from build123d import *

# Parameters (mm, degrees)
F0_R     = 11
F0_R_2   = 9.25
F1_DEPTH = 10
F3_DEPTH = 6
F4_SIZE  = 0.99999


# Not quite as in the source:
# - a fillet or chamfer is up to 0.001 mm smaller than in the source, because OpenCascade refuses the exact size


with BuildPart() as f1:
    # F0 (on Top) → F1 (new body)
    with BuildSketch(Plane.XY):
        Circle(F0_R)
        Circle(F0_R_2, mode=Mode.SUBTRACT)
    extrude(amount=F1_DEPTH)

    # F2 (on face) → F3 (cut)
    with BuildSketch(Plane.XY.offset(10)):
        with BuildLine():
            Line((-10, -4.582575695), (-10, 4.582575695))
            ThreePointArc((-10, 4.582575695), (-11, 0), (-10, -4.582575695))
        make_face()
        with BuildLine():
            ThreePointArc((11, 0), (10.7470926301, 2.3452078799), (10, 4.582575695))
            Line((10, 4.582575695), (10, -4.582575695))
            ThreePointArc((10, -4.582575695), (10.7470926301, -2.3452078799), (11, 0))
        make_face()
    extrude(amount=-F3_DEPTH, mode=Mode.SUBTRACT)

    # F4 (size 1 in the source; OpenCascade refuses exactly that, so slightly less here)
    f4_edges = [f1.edges().sort_by_distance(p)[0] for p in [
        (-11, 0, 0),
        (0, -11, 10),
        (0, 11, 10),
    ]]
    chamfer(f4_edges, length=F4_SIZE)


solid = f1.part
Build history of the part. All positions in model axes, mm. A direction names the side the tool comes from. Round coordinates to 2 decimals unless told otherwise and drop trailing zeros. Write each loop counter-clockwise with the first axis right and the second up, starting at its lowest first coordinate (ties: lowest second). Pieces come first, ordered by that corner, then holes. Notation, with made-up numbers: M 2,69 L 32,69 A23 cw 32,106 Z; hole C 25,74.5 d10. An arc over 180 degrees is marked long. Answer in a Markdown table with one row per item.
1. Saw through at A-A (z = 6.25). List the corners of the cut face in (x, y).
Geometry check:
| item | result |
|---|---|
| outline | M -10,-4.58 A11 ccw 10,-4.58 L 10,4.58 A11 ccw -10,4.58 Z; hole C 0,0 d18.5 |
2. Which spindle directions (+Z, -Z, +X, -X, +Y, -Y) get a long thin tool onto all of the face, cutting with end or side? Do faces 5 (the face through (-11, 0, 3)), 6 (the face through (10, 0, 7)), 7 (the face through (-10.4, 0.1, 4)). Say none if no direction does.
Geometry check:
| item | result |
|---|---|
| face 5 | +Z, -Z |
| face 6 | +Z, +X, +Y, -Y |
| face 7 | +Z, -X, +Y, -Y |
3. Probe L1, parallel to Y at x = 0, z = 6; L2, parallel to Y at x = 2.5, z = 8.5; L3, parallel to X at y = 1.75, z = 0.5. List the from-to ranges inside material, lowest first. Write a range as [from, to].
Geometry check:
| item | result |
|---|---|
| L1 | [-11, -9.25], [9.25, 11] |
| L2 | [-10.71, -8.91], [8.91, 10.71] |
| L3 | [-10.35, -9.08], [9.08, 10.35] |
4. Mould opens along X. For faces 1 (the face through (-0.2, -10.2, 9.8)), 2 (the face through (-10, 0, 7)), 3 (the face through (9, -3, 10)), 4 (the face through (-2.01, -9.03, 4.93)) say: +X half, -X half, draft (parallel to the pull), parting line (faces both ways), or undercut.
Geometry check:
| item | result |
|---|---|
| face 1 | parting line |
| face 2 | -X half |
| face 3 | draft |
| face 4 | undercut |
5. Saw through at C-C (z = 3.5). List the corners of the cut face in (x, y).
Geometry check:
| item | result |
|---|---|
| outline | C 0,0 d22; hole C 0,0 d18.5 |
6. Saw through at B-B (x = 0). List the corners of the cut face in (y, z), and give its area (3 significant figures).
Geometry check:
| item | result |
|---|---|
| outline | M -11,1 L -10,0 L -9.25,0 L -9.25,10 L -10,10 L -11,9 Z; M 9.25,0 L 10,0 L 11,1 L 11,9 L 10,10 L 9.25,10 Z |
| area | 33.0 mm2 |
7. Flat gauge pins, fed straight in: P1, Ø0.5, axis at x = 10.5, y = -1.5, coming from the +Z side; P2, Ø2, axis at y = 2, z = 2, coming from the -X side; P3, Ø1.1, axis at x = -10.5, y = -1.5, coming from the +Z side. Where does each tip first touch, or does it go through?
Geometry check:
| item | result |
|---|---|
| P1 | z = 4 |
| P2 | x = -10.95 |
| P3 | z = 9.94 |
